```python
from build123d import *

# Parameters (mm, degrees)
F0_W     = 12.7
F0_H     = 10.16
F1_DEPTH = 1.27
F3_DEPTH = 1.27
F4_R     = 0.3175
F5_R     = 0.3175
F6_R     = 0.508
F7_DEPTH = 7.62
F8_R     = 0.508
F9_DEPTH = 7.62


with BuildPart() as f1:
    # F0 (on Top) → F1 (new body)
    with BuildSketch(Plane.XY):
        with Locations((6.35, -5.08)):
            Rectangle(F0_W, F0_H)
    extrude(amount=F1_DEPTH)

    # F2 (on face) → F3 (join)
    with BuildSketch(Plane.XY.offset(1.27)):
        Polygon((4.682481, -5.194736), (3.598544, -2.897633), (2.265116, -5.059477), (3.349053, -7.356579), align=None)
        Polygon((7.538687, -5.274285), (8.856249, -7.445835), (10.158128, -5.264846), (8.840566, -3.093297), align=None)
    extrude(amount=F3_DEPTH)

    # F4
    f4_edges = [f1.edges().sort_by_distance(p)[0] for p in [
        (3.349053, -7.356579, 1.905),
        (8.856249, -7.445835, 1.905),
    ]]
    fillet(f4_edges, radius=F4_R)

    # F5
    f5_edges = [f1.edges().sort_by_distance(p)[0] for p in [
        (7.538687, -5.274285, 1.905),
        (2.265116, -5.059477, 1.905),
        (3.598544, -2.897633, 1.905),
        (8.840566, -3.093297, 1.905),
        (10.158128, -5.264846, 1.905),
        (4.682481, -5.194736, 1.905),
    ]]
    fillet(f5_edges, radius=F5_R)

    # F6 (on face) → F7 (join)
    with BuildSketch(Plane.XY.offset(2.54)):
        with Locations((3.498474, -4.265051)):
            Circle(F6_R)
    extrude(amount=F7_DEPTH)

    # F8 (on face) → F9 (join)
    with BuildSketch(Plane.XY.offset(2.54)):
        with Locations((8.828444, -4.307084)):
            Circle(F8_R)
    extrude(amount=F9_DEPTH)


solid = f1.part
```
Geometry check sheet. Reference: the model listing, model coordinates, mm. A direction names the side the tool comes from. Coordinates: 2 decimals unless noted, no trailing zeros. Write each loop counter-clockwise with the first axis right and the second up, starting at its lowest first coordinate (ties: lowest second). Pieces come first, ordered by that corner, then holes. Notation, with made-up numbers: M 31,-29.75 L 64,-29.75 A9 ccw 64,-16.75 Z; hole C 84.5,37.25 d5. An arc over 180 degrees is marked long. Use one line per item in the form item = value. Start each with the question number.
1) Section check D-D on x = 5.5. Enter the section's corners in (y, z).
2) Release check for a two-part mould opening along X. For faces 6 (the flat face through (3.5, -4.3, 10.16)), 7 (the flat face through (8.11, -4.32, 1.9)), 8 (the flat face through (0, -5, 1)) record: pulls with the +X half, pulls with the -X half, needs draft (parallel to the pull), parting line crosses it, or undercut.
3) Section check C-C on y = -8.25. Enter the section's corners in (x, z), and give its area (3 significant figures).
4) Go/stop test with flat-tipped pins: pin 1 Ø4 at (y, z) = (-6.5, 8.5) entering from +X; pin 2 Ø4 at (x, z) = (10, 3.5) entering from +Y; pin 3 Ø3 at (x, y) = (11, -3) entering from +Z. Record where each tip stops, or that it passes through.
5) Set-up check for faces 1 (the flat face through (2.83, -4.14, 1.9)), 2 (the flat face through (4.23, -4.24, 1.9)), 3 (the flat face through (4.12, -6.11, 1.9)), 4 (the flat face through (2.714, -6.01, 1.896)), 5 (the flat face through (6, -5, 1.27)): record each of +Z, -Z, +X, -X, +Y, -Y from which the full face is reachable in a straight line by a thin tool's end or side.
6) Thickness scan on probe 1 along Z at (x, y) = (4.75, -6); probe 2 along Z at (x, y) = (10, -5.25); probe 3 along Y at (x, z) = (3.5, 7.75). Record the ranges inside material, lowest first. Write a range as from..to.
7) Section check B-B on x = 8. Enter the section's corners in (y, z), and give its area (3 significant figures).
Responses:
q1.outline = M -10.16,0 L 0,0 L 0,1.27 L -10.16,1.27 Z
q2.face_6 = needs draft
q2.face_7 = undercut
q2.face_8 = pulls with the -X half
q3.outline = M 0,0 L 12.7,0 L 12.7,1.27 L 0,1.27 Z
q3.area = 16.1 mm2
q4.pin_1 = 9.3
q4.pin_2 = -3.39
q4.pin_3 = 1.27
q5.face_1 = +Z, -X, +Y
q5.face_2 = +Z, +Y
q5.face_3 = +Z, -Y
q5.face_4 = +Z, -X, -Y
q5.face_5 = +Z
q6.probe_1 = 0..1.27
q6.probe_2 = 0..2.54
q6.probe_3 = -4.77..-3.76
q7.outline = M -10.16,0 L 0,0 L 0,1.27 L -4.5,1.27 L -4.5,2.54 L -6.03,2.54 L -6.03,1.27 L -10.16,1.27 Z
q7.area = 14.9 mm2
